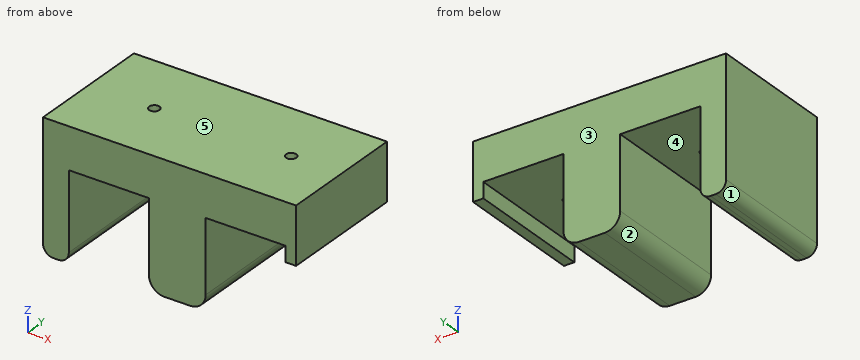
from build123d import *

# Parameters (mm, degrees)
BOSS_EXTRUDE1_DEPTH = 25
FILLET2_R           = 3
FILLET3_R           = 2
SKETCH3_R           = 1
CUT_EXTRUDE1_DEPTH  = 58.576036682


with BuildPart() as part:
    # Sketch1 → Boss-Extrude1 (new body)
    with BuildSketch(Plane(origin=(0, 0, 0), x_dir=(1, 0, 0), z_dir=(0, 1, 0))):
        Polygon((0, 0), (49, 0), (49, 11), (47, 11), (47, 8), (31.5, 8), (31.5, 25), (20.5, 25), (20.5, 8), (5, 8), (5, 25), (0, 25), align=None)
    extrude(amount=BOSS_EXTRUDE1_DEPTH)

    # Fillet2
    fillet2_edges = [part.edges().sort_by_distance(p)[0] for p in [
        (20.5, 12.5, -25),
        (31.5, 12.5, -25),
    ]]
    fillet(fillet2_edges, radius=FILLET2_R)

    # Fillet3
    fillet3_edges = [part.edges().sort_by_distance(p)[0] for p in [
        (0, 12.5, -25),
        (5, 12.5, -25),
    ]]
    fillet(fillet3_edges, radius=FILLET3_R)

    # Sketch3 → Cut-Extrude1 (cut, through all)
    with BuildSketch(Plane(origin=(0, 0, -8), x_dir=(-1, 0, 0), z_dir=(0, 0, -1))):
        with Locations((-39.25, 12.5)):
            Circle(SKETCH3_R)
        with Locations((-12.75, 12.5)):
            Circle(SKETCH3_R)
    extrude(amount=-CUT_EXTRUDE1_DEPTH, mode=Mode.SUBTRACT)


solid = part.part
Here's how the part is built. I have some questions about the finished solid (model axes, mm). Face numbers are marked on the shaded views. A direction names the side the tool comes from. Give positions to 0.01 mm unless a question says otherwise; leave off trailing zeros. Order: outer loops, then holes, each group sorted by start corner. A loop starts at its lowest first (then second) coordinate and runs counter-clockwise, first axis right, second up. Notation, with made-up numbers: (-32.75, -32) -> (-25.75, -32) arc R7 cw to (-25.75, -26) -> close; hole circle Ø10 at (38, 21). An arc over 180 degrees is marked (long way). One line per item, written item: value. Start each with the question number.
1. Imagine slicing it at D-D, the plane x = 43. List the corners of the cut face in (y, z) for me, plus the area to 3 significant figures.
2. For the marked faces 4 and 5, which set-ups out of +Z, -Z, +X, -X, +Y, -Y let a thin tool reach every point of the face, with its end or its side?
3. Imagine slicing it at A-A, the plane z = -11.75. List the corners of the cut face in (x, y) for me.
4. Will these pins go through, and if not, where does the flat tip stop? pin 1 Ø4.5 at (x, y) = (14, 6.5) entering from -Z; pin 2 Ø7.5 at (y, z) = (15, -19) entering from +X; pin 3 Ø10 at (x, y) = (32.5, 5.5) entering from +Z; pin 4 Ø0.6 at (x, y) = (48, 7.5) entering from -Z.
5. Imagine slicing it at C-C, the plane y = 23.25. List the corners of the cut face in (x, z) for me, plus the area to 3 significant figures.
6. Imagine slicing it at B-B, the plane x = 12.75. List the corners of the cut face in (y, z) for me, plus the area to 3 significant figures.
7. I need wall thicknesses on probe 1 along X at (y, z) = (11.5, -16); probe 2 along Y at (x, z) = (39.25, -4.5); probe 3 along X at (y, z) = (13, -4.5). Which ranges of each line are inside material? Lowest first, please. Write a range as from..to.
8. We'd pull the mould along X, two halves only. Please class the marked faces 1, 2 and 3: released by +X, released by -X, zero draft, split by the parting line, or undercut.
Values follow:
1. outline: (0, -8) -> (25, -8) -> (25, 0) -> (0, 0) -> close
1. area: 200 mm2
2. face 4: -Z, +Y, -Y
2. face 5: +Z, +X, -X, +Y, -Y
3. outline: (0, 0) -> (5, 0) -> (5, 25) -> (0, 25) -> close; (20.5, 0) -> (31.5, 0) -> (31.5, 25) -> (20.5, 25) -> close
4. pin 1: stops at z = -8
4. pin 2: stops at x = 31.5
4. pin 3: stops at z = 0
4. pin 4: stops at z = -11
5. outline: (0, -23) arc R2 ccw to (2, -25) -> (3, -25) arc R2 ccw to (5, -23) -> (5, -8) -> (20.5, -8) -> (20.5, -22) arc R3 ccw to (23.5, -25) -> (28.5, -25) arc R3 ccw to (31.5, -22) -> (31.5, -8) -> (47, -8) -> (47, -11) -> (49, -11) -> (49, 0) -> (0, 0) -> close
5. area: 664 mm2
6. outline: (0, -8) -> (11.5, -8) -> (11.5, 0) -> (0, 0) -> close; (13.5, -8) -> (25, -8) -> (25, 0) -> (13.5, 0) -> close
6. area: 184 mm2
7. probe 1: x = 0..5, 20.5..31.5
7. probe 2: y = 0..11.5, 13.5..25
7. probe 3: x = 0..11.88, 13.62..38.38, 40.12..49
8. face 1: released by -X
8. face 2: undercut
8. face 3: zero draft
